The listing builds one solid part. Answer for the finished solid, in the listing's coordinates (mm). A direction names the side the tool comes from. Coordinates: 2 decimals unless noted, no trailing zeros. Loops run counter-clockwise (first coordinate to the right, second up) from the corner with the lowest first, then second, coordinate; pieces in that order, holes last. Notation, with made-up numbers: (24.25, -16) - (70.25, -16) arc R33 cw to (70.25, 12) - close; hole circle Ø7 at (7.25, 24.5). An arc over 180 degrees is marked (long way). Put each result on its own line as item: value.
```python
from build123d import *

# Parameters (mm, degrees)
F0_R     = 6.35
F1_DEPTH = 12.7
F2_R     = 1.651
F3_DEPTH = 12.7
F4_R     = 1.647045
F5_DEPTH = 3.302


with BuildPart() as f1:
    # F0 (on Top) → F1 (new body)
    with BuildSketch(Plane.XY):
        with Locations((-24.937442, 17.330116)):
            Circle(F0_R)
    extrude(amount=-F1_DEPTH)

    # F2 (on Top) → F3 (join)
    with BuildSketch(Plane.XY):
        with Locations((-24.937442, 17.330116)):
            Circle(F2_R)
    extrude(amount=F3_DEPTH)

    # F4 (on face) → F5 (join)
    with BuildSketch(Plane(origin=(0, 0, -12.7), x_dir=(1, 0, 0), z_dir=(0, 0, -1))):
        with Locations((-24.937442, -17.330116)):
            Circle(F4_R)
    extrude(amount=F5_DEPTH)


solid = f1.part
```
1) Each of these flat-tipped pins is pushed along its axis until it touches: pin 1 (2 mm diameter, centred on x = -30, y = 22, fed in from +Z); pin 2 (1.5 mm diameter, centred on x = -28.5, z = 9.5, fed in from -Y); pin 3 (3 mm diameter, centred on x = -21.5, z = -9, fed in from +Y); pin 4 (6 mm diameter, centred on y = 14.5, z = 8.5, fed in from -X). Where does it stop, or does it pass through?
Found:
pin 1: stops at z = 0
pin 2: passes through
pin 3: stops at y = 23.38
pin 4: stops at x = -26.59
2) The part is cut by section B-B (y = 16.25). Give the vertices of the cut face in (x, z).
Found:
outline: (-31.19, -12.7) - (-26.18, -12.7) - (-26.18, -16) - (-23.69, -16) - (-23.69, -12.7) - (-18.68, -12.7) - (-18.68, 0) - (-23.69, 0) - (-23.69, 12.7) - (-26.19, 12.7) - (-26.19, 0) - (-31.19, 0) - close
3) The part is cut by section C-C (z = -13.5). Give the vertices of the cut face in (x, y).
Found:
outline: circle Ø3.29 at (-24.94, 17.33)
4) For faces 1 (the face through (-25, 17, -16.002)), 2 (the face through (-23.363, 17.826, 6.261)), 3 (the face through (-23.6, 16, -12.7)), determine the directions among +Z, -Z, +X, -X, +Y, -Y from which every point of the face is accessible in a straight line to the end or side of a thin tool.
Found:
face 1: -Z, +X, -X, +Y, -Y
face 2: +Z
face 3: -Z
5) The part is cut by section A-A (x = -25.5). Give the vertices of the cut face in (y, z), and give its area (3 significant figures).
Found:
outline: (11.01, -12.7) - (15.78, -12.7) - (15.78, -16) - (18.88, -16) - (18.88, -12.7) - (23.66, -12.7) - (23.66, 0) - (18.88, 0) - (18.88, 12.7) - (15.78, 12.7) - (15.78, 0) - (11.01, 0) - close
area: 210 mm^2
6) Straight lines are drawn through the part: L1, parallel to Z at x = -26.25, y = 20.5; L2, parallel to X at y = 17.5, z = -4.75; L3, parallel to Y at x = -21, z = -8. For each, find the intervals that lie inside material, in ascending order. Write a range as [from, to].
Found:
L1: z = [-12.7, 0]
L2: x = [-31.29, -18.59]
L3: y = [12.35, 22.31]
7) The part is cut by section D-D (y = 13.25). Give the vertices of the cut face in (x, z).
Found:
outline: (-29.8, -12.7) - (-20.07, -12.7) - (-20.07, 0) - (-29.8, 0) - close
